Can you work these out from the drawing? Everything is in mm from the part's minimum corner. Round coordinates to 2 decimals unless told otherwise and drop trailing zeros. Write each loop counter-clockwise with the first axis right and the second up, starting at its lowest first coordinate (ties: lowest second). Pieces come first, ordered by that corner, then holes. Notation, with made-up numbers: (34.5, -33) - (59.5, -33) arc R20 cw to (59.5, 4) - close; hole circle Ø2 at (-5.75, 64.25). An arc over 180 degrees is marked (long way). One line per item, written item: value. Start each with the question number.
(1) I want a section at A-A on z = 7.62. List the corners of the cut face in (x, y) for me, plus the area to 3 significant figures.
(2) Thinking about a two-plate mould opening in X: for the marked faces 1 and 2, which applies, +X half, -X half, draft (parallel to the pull), parting line (faces both ways), or undercut?
(3) I want a section at B-B on x = 93.98. List the corners of the cut face in (y, z) for me, plus the area to 3 significant figures.
(4) I want a section at C-C on y = 2.9. List the corners of the cut face in (x, z) for me.
(5) If I drill on L1, parallel to Z at x = 93.98, y = 0.45; L2, parallel to X at y = 0.4, z = 53.34; L3, parallel to X at y = 2.9, z = 21.5, over which ranges is the centre line in solid material (lowest first)? Write a range as from..to.
(6) I want a section at D-D on x = 64.5. List the corners of the cut face in (y, z) for me, plus the area to 3 significant figures.
(7) I'm going to push flat-ended pins straight in: pin 1 Ø1.2 at (x, z) = (93.98, 7.62) entering from -Y; pin 2 Ø8 at (x, z) = (81.5, 33) entering from +Y. Where does each tip first touch, or does it pass through?
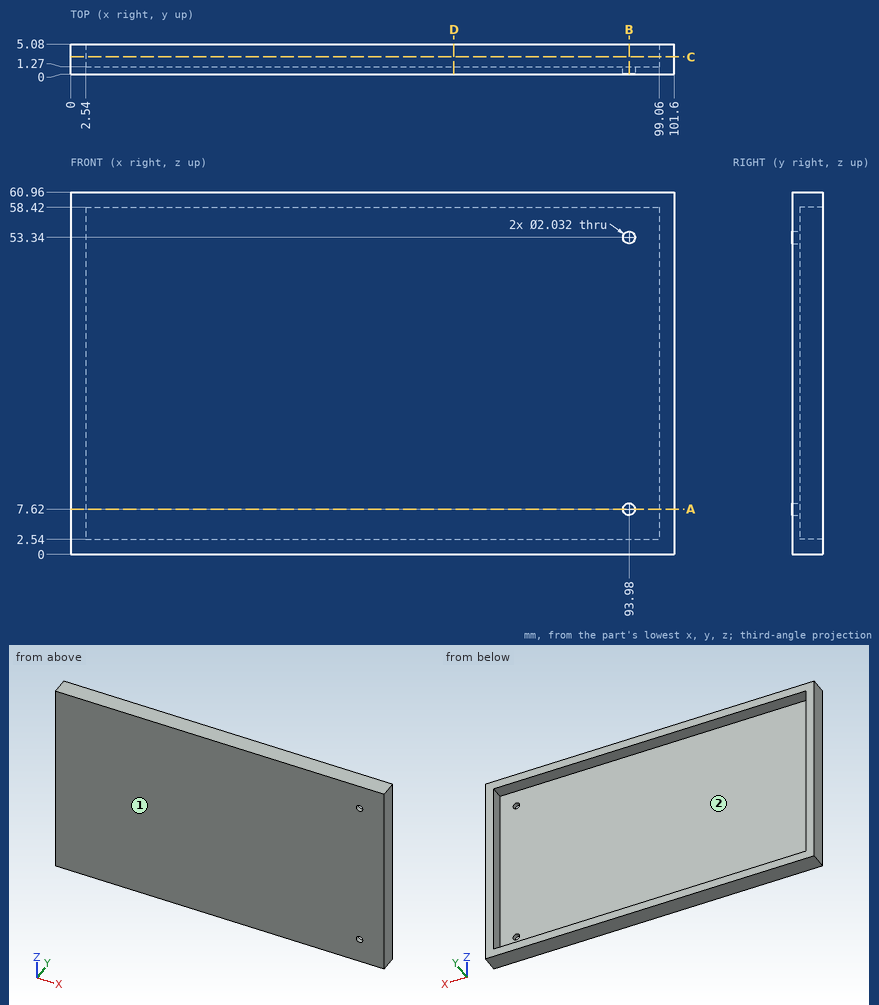
Established:
1. outline: (0, 0) - (92.96, 0) - (92.96, 1.27) - (2.54, 1.27) - (2.54, 5.08) - (0, 5.08) - close; (95, 0) - (101.6, 0) - (101.6, 5.08) - (99.06, 5.08) - (99.06, 1.27) - (95, 1.27) - close
1. area: 146 mm2
2. face 1: draft
2. face 2: undercut
3. outline: (0, 0) - (5.08, 0) - (5.08, 2.54) - (1.27, 2.54) - (1.27, 6.6) - (0, 6.6) - close; (0, 8.64) - (1.27, 8.64) - (1.27, 52.32) - (0, 52.32) - close; (0, 54.36) - (1.27, 54.36) - (1.27, 58.42) - (5.08, 58.42) - (5.08, 60.96) - (0, 60.96) - close
3. area: 91.6 mm2
4. outline: (0, 0) - (101.6, 0) - (101.6, 60.96) - (0, 60.96) - close; hole (2.54, 2.54) - (99.06, 2.54) - (99.06, 58.42) - (2.54, 58.42) - close
5. L1: 0..6.6, 8.64..52.32, 54.36..60.96
5. L2: 0..92.96, 95..101.6
5. L3: 0..2.54, 99.06..101.6
6. outline: (0, 0) - (5.08, 0) - (5.08, 2.54) - (1.27, 2.54) - (1.27, 58.42) - (5.08, 58.42) - (5.08, 60.96) - (0, 60.96) - close
6. area: 96.8 mm2
7. pin 1: through
7. pin 2: y = 1.27
